from build123d import *

# Parameters (mm, degrees)
F1_ANGLE = 180


# Not quite as in the source:
# - the dataset's text gives a spline's control points without its knots; the knots are read off the source's solid


with BuildPart() as f1:
    # F0 (on Top) → F1 (revolve)
    with BuildSketch(Plane.XY):
        with BuildLine():
            Line((-15.0155171111, 69.1660211089), (-41.8962485401, 69.1660211089))
            Line((-41.8962485401, 69.1660211089), (-41.8963717975, 59.1659390384))
            Line((-41.8963717975, 59.1659390384), (-20.2472324434, 59.1659390491))
            add(Edge.make_bspline(
                [(33.1035238522, -71.9149671498), (32.1956039275, -68.8975063653), (30.6294745703, -63.7909684), (28.3196130402, -56.4725000911), (26.2505964512, -50.0519807984), (24.0990817026, -43.5000705854), (21.8647786098, -36.8081776409), (19.5529594243, -30.0145868681), (16.3683569347, -20.8591029876), (12.2012714526, -9.3103100361), (6.9186898701, 4.4674267501), (-0.4742289291, 22.3935878339), (-8.3508677217, 39.1456078716), (-15.719087441, 52.1661135478), (-19.0226095104, 57.3411254378), (-20.2472324434, 59.1659390491)],
                knots=[0.3286112864, 0.3286112864, 0.3286112864, 0.3286112864, 0.375, 0.40625, 0.4375, 0.46875, 0.5, 0.53125, 0.5625, 0.625, 0.6875, 0.75, 0.875, 0.9375, 0.9742015542, 0.9742015542, 0.9742015542, 0.9742015542], degree=3))
            Line((33.1035238522, -71.9149671498), (42.9852085247, -71.9149671498))
            add(Edge.make_bspline(
                [(42.9852085247, -71.9149671498), (39.9590182528, -62.0062274912), (25.1654617563, -16.1855840824), (4.2573580541, 42.5444841716), (-15.0155171111, 69.1660211089)],
                knots=[0.3152642845, 0.3152642845, 0.3152642845, 0.3152642845, 0.4687726258, 1, 1, 1, 1], degree=3))
        make_face()
        with BuildLine():
            add(Edge.make_bspline(
                [(58.1037514599, -130.8339788911), (54.1906296951, -111.0809956414), (49.2001783618, -92.2648171488), (42.9852085247, -71.9149671498)],
                knots=[0, 0, 0, 0, 0.3152642845, 0.3152642845, 0.3152642845, 0.3152642845], degree=3))
            Line((42.9852085247, -71.9149671498), (33.1035238522, -71.9149671498))
            add(Edge.make_bspline(
                [(48.1037514599, -130.8339788911), (46.7078713802, -123.9406660172), (44.3454121428, -113.2929426353), (40.6901923565, -98.7187159107), (37.5318209869, -87.037434), (34.9410521612, -78.0565994752), (33.4188539578, -72.9629629054), (33.1035238522, -71.9149671498)],
                knots=[0.0128290388, 0.0128290388, 0.0128290388, 0.0128290388, 0.125, 0.1875, 0.25, 0.3125, 0.3286112864, 0.3286112864, 0.3286112864, 0.3286112864], degree=3))
            Line((48.1037514599, -130.8339788911), (58.1037514599, -130.8339788911))
        make_face()
    revolve(axis=Axis((-41.8963717672, -2.0099732555, 0), (5e-10, -1, 0)), revolution_arc=F1_ANGLE)


solid = f1.part
Geometry check sheet. Reference: the model listing, model coordinates, mm. Give positions to 0.01 mm unless a question says otherwise; leave off trailing zeros. Answer as CSV lines item,"result". Start each with the question number.
Q1. Release check for a two-part mould opening along X. For faces 1 (the face through (19, -23, 0)), 2 (the face through (-42, 59.166, 9)) record: pulls with the +X half, pulls with the -X half, needs draft (parallel to the pull), parting line crosses it, or undercut.
Q2. Material ranges on L1, parallel to X at y = 11, z = 21; L2, parallel to X at y = -40.5, z = 14.5; L3, parallel to Z at x = -22.5, y = -104, recorded low to high.
Q3. Go/stop test with flat-tipped pins: pin 1 (1 mm diameter, centred on x = -70.5, y = -105, fed in from -Z); pin 2 (2 mm diameter, centred on y = -33, z = 27.5, fed in from +X); pin 3 (1.5 mm diameter, centred on x = -13, y = -45, fed in from -Z). Record where each tip stops, or that it passes through.
Geometry says:
1,face 1,"needs draft"
1,face 2,"undercut"
2,L1,"-94.24 to -82.94, -0.85 to 10.45"
2,L2,"-115.29 to -105.25, 21.46 to 31.5"
2,L3,"81.63 to 91.9"
3,pin 1,"z = 78.92"
3,pin 2,"x = 25.52"
3,pin 3,"z = 59.42"
